from build123d import *

# Parameters (mm, degrees)
F0_W     = 15.6
F0_H     = 5
F1_DEPTH = 40
F2_R     = 1
F3_R     = 1
F8_D     = 2.2606
F10_D    = 2.2606


# Not quite as in the source:
# - a feature of the source that left no trace in its solid (it failed there, or was rolled back) is left out


with BuildPart() as f1:
    # F0 (on Front) → F1 (new body, symmetric)
    with BuildSketch(Plane.XZ):
        with Locations((0, 5.57)):
            Rectangle(F0_W, F0_H)
    extrude(amount=F1_DEPTH, both=True)

    # F2
    f2_edges = [f1.edges().sort_by_distance(p)[0] for p in [
        (7.8, 0, 8.07),
    ]]
    fillet(f2_edges, radius=F2_R)

    # F3
    f3_edges = [f1.edges().sort_by_distance(p)[0] for p in [
        (-7.8, 0, 8.07),
    ]]
    fillet(f3_edges, radius=F3_R)

    # F8 (through all)
    with Locations(Plane(origin=(0, 0, 0), x_dir=(1, 0, 0), z_dir=(0, 0, -1))):
        with Locations((0, 35)):
            Hole(F8_D / 2)

    # F10 (through all)
    with Locations(Plane(origin=(0, 0, 0), x_dir=(1, 0, 0), z_dir=(0, 0, -1))):
        with Locations((0, -35)):
            Hole(F10_D / 2)


solid = f1.part
Design review of the part built by this model. Coordinates are the model's own, in mm. Coordinates: 2 decimals unless noted, no trailing zeros. Loops run counter-clockwise (first coordinate to the right, second up) from the corner with the lowest first, then second, coordinate; pieces in that order, holes last. Notation, with made-up numbers: (70.25, 17.5) -> (75.25, 17.5) arc R26 ccw to (75.25, 46.5) -> close; hole circle Ø3 at (4, 58.5). An arc over 180 degrees is marked (long way). Use a Markdown table: item, result. Add a question column.
Item 1: We need section A-A, the plane x = 0. Write out the cut boundary in (y, z).
Item 2: We need section B-B, the plane y = -35. Write out the cut boundary in (x, z), and give its area (3 significant figures).
Item 3: Wall thickness on L1, parallel to Y at x = 0, z = 5.6; L2, parallel to X at y = -35, z = 4.6; L3, parallel to Y at x = -0.75, z = 6.95: over which ranges is each line inside the solid? List them lowest first. Write a range as from..to.
Item 4: Clearance check with a flat-ended pin moving along its axis: P1, Ø1.4, axis at x = 0, y = 35, coming from the +Z side. State where the tip first meets the part, or that it passes through.
Item 5: The part is to be moulded in two halves that separate along Y. For faces 1 (the flat face through (0, -40, 6)), 2 (the cylindrical face through (0.15, 33.88, 5.61)), 3 (the flat face through (0, -1, 8.07)), say which applies: +Y half, -Y half, draft (parallel to the pull), parting line (faces both ways), or undercut.
Numbers:
| question | item | result |
|---|---|---|
| 1 | outline | (-40, 3.07) -> (-36.13, 3.07) -> (-36.13, 8.07) -> (-40, 8.07) -> close; (-33.87, 3.07) -> (33.87, 3.07) -> (33.87, 8.07) -> (-33.87, 8.07) -> close; (36.13, 3.07) -> (40, 3.07) -> (40, 8.07) -> (36.13, 8.07) -> close |
| 2 | outline | (-7.8, 3.07) -> (-1.13, 3.07) -> (-1.13, 8.07) -> (-6.8, 8.07) arc R1 ccw to (-7.8, 7.07) -> close; (1.13, 3.07) -> (7.8, 3.07) -> (7.8, 7.07) arc R1 ccw to (6.8, 8.07) -> (1.13, 8.07) -> close |
| 2 | area | 66.3 mm^2 |
| 3 | L1 | y = -40..-36.13, -33.87..33.87, 36.13..40 |
| 3 | L2 | x = -7.8..-1.13, 1.13..7.8 |
| 3 | L3 | y = -40..-35.85, -34.15..34.15, 35.85..40 |
| 4 | P1 | passes through |
| 5 | face 1 | -Y half |
| 5 | face 2 | undercut |
| 5 | face 3 | draft |
